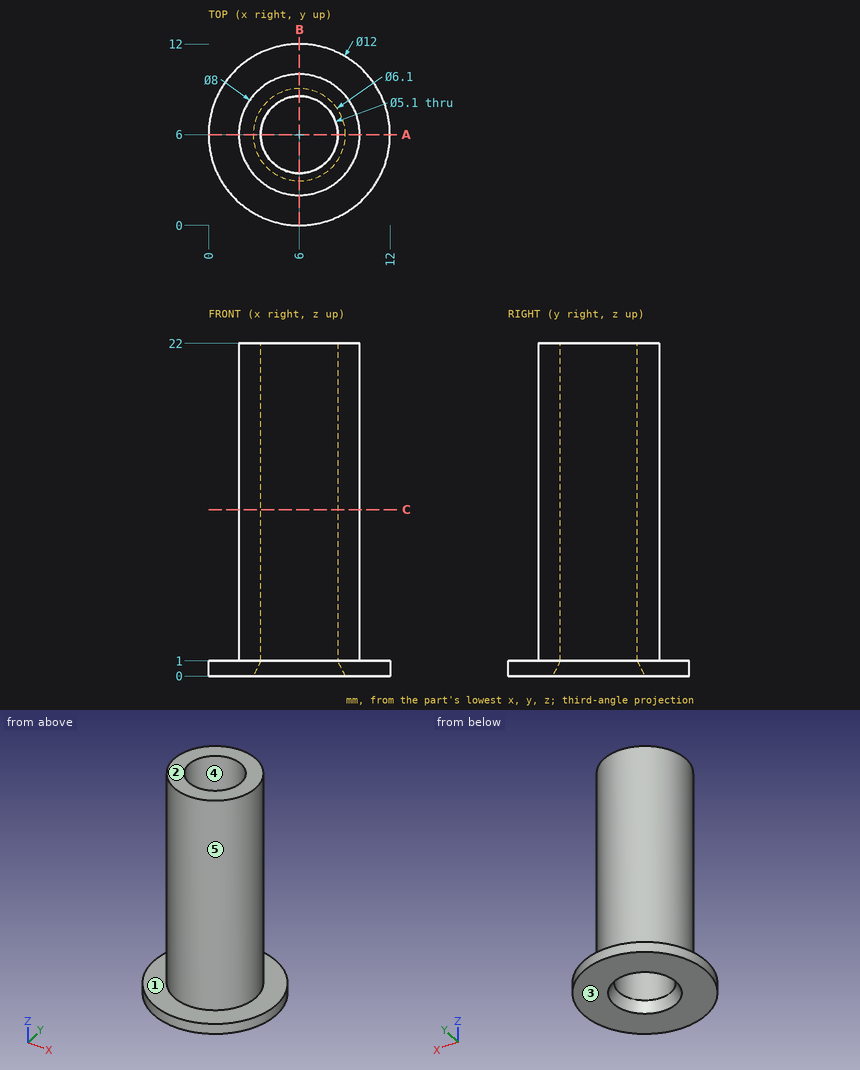
For this review, use the dimensioned drawing (mm, ordinates from the lowest corner) and the shaded views. A direction names the side the tool comes from. Coordinates: 2 decimals unless noted, no trailing zeros. Loops run counter-clockwise (first coordinate to the right, second up) from the corner with the lowest first, then second, coordinate; pieces in that order, holes last.
1. Add section C-C, the plane z = 11. Give the boundary of the cut face in (x, y).
2. Add section A-A, the plane y = 6. Give the boundary of the cut face in (x, z), then the cut area to 3 significant figures.
3. Insertion check: P1, Ø6, axis at x = 3.5, z = 18, coming from the +Y side; P2, Ø6, axis at y = 8, z = 15.5, coming from the +X side; P3, Ø1, axis at x = 3.5, z = 4, coming from the -Y side. Each pin has a flat end and moves straight along its axis. Give the tip position at first contact, or say it passes through.
4. Mouldability with a two-part tool opening along Y and no side actions: class the marked faces 3, 4 and 5 as +Y half, -Y half, draft (parallel to the pull), parting line (faces both ways), or undercut.
5. For line 1 (Y direction, x = 6, z = 16.5); line 2 (Z direction, x = 10.5, y = 7.5); line 3 (Y direction, x = 7.25, z = 20.25), list the stretches that pass through material, from the lowest coordinate up.
6. For the marked faces 1 and 2, list the 3-axis set-ups (+Z, -Z, +X, -X, +Y, -Y) from which the entire face can be reached by the end or side of a thin tool; tool diameter is ignored.
Result:
1. outline: circle Ø8 at (6, 6); hole circle Ø5.1 at (6, 6)
2. outline: (0, 0) - (2.95, 0) - (3.45, 1) - (3.45, 22) - (2, 22) - (2, 1) - (0, 1) - close; (8.55, 1) - (9.05, 0) - (12, 0) - (12, 1) - (10, 1) - (10, 22) - (8.55, 22) - close
2. area: 67.3 mm2
3. P1: stops at y = 10
3. P2: stops at x = 10
3. P3: stops at y = 2.54
4. face 3: draft
4. face 4: undercut
4. face 5: parting line
5. line 1: y = 2 to 3.45, 8.55 to 10
5. line 2: z = 0 to 1
5. line 3: y = 2.2 to 3.78, 8.22 to 9.8
6. face 1: +Z
6. face 2: +Z, +X, -X, +Y, -Y
